Design review of the part built by this model. Coordinates are the model's own, in mm. Give positions to 0.01 mm unless a question says otherwise; leave off trailing zeros. Order: outer loops, then holes, each group sorted by start corner. A loop starts at its lowest first (then second) coordinate and runs counter-clockwise, first axis right, second up.
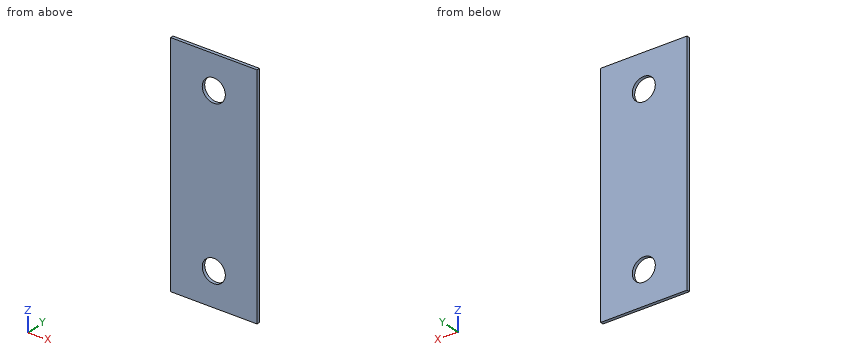
Autodesk Inventor part; units mm, degrees
ref_plane "YZ Plane" through (0, 0, 0) normal (1, 0, 0) x (0, 1, 0)
ref_plane "XZ Plane" through (0, 0, 0) normal (0, 1, 0) x (-1, 0, 0)
ref_plane "XY Plane" through (0, 0, 0) normal (0, 0, 1) x (1, 0, 0)
sketch "Sketch1" plane through (0, 0, 0) normal (0, 1, 0) x (-1, 0, 0)
  line L0 (0, 0) -> (19.05, 0)
  line L1 (19.05, 0) -> (19.05, -50.8)
  line L2 (19.05, -50.8) -> (0, -50.8)
  line L3 (0, -50.8) -> (0, 0)
  line L4 (19.05, 0) -> (0, 0)
  line L5 (0, 0) -> (0, -14.732)
  line L6 (0, -14.732) -> (19.05, -14.732)
  line L7 (19.05, -14.732) -> (19.05, 0)
  line L8 (19.05, -50.8) -> (0, -50.8)
  line L9 (0, -50.8) -> (0, -36.068)
  line L10 (0, -36.068) -> (19.05, -36.068)
  line L11 (19.05, -36.068) -> (19.05, -50.8)
  circle A0 centre (9.525, -7.366) radius 2.54
  circle A1 centre (9.525, -43.434) radius 2.54
  dimension "d0" = 50.8
  dimension "d1" = 19.05
  dimension "d2" = 14.732
  dimension "d3" = 14.732
  dimension "d4" = 5.08
  dimension "d5" = 5.08
extrude "Extrusion1" add sketch "Sketch1" along normal blind 0.7
equation "\"d3\" = d2"
properties part number "Part18.iptMotorProtector2"
1. Take a section at B-B (x = -8). State the section outline as (y, z) points, then the cut area to 3 significant figures.
Recorded:
outline: (0, -50.8) - (0.7, -50.8) - (0.7, -45.47) - (0, -45.47) - close; (0, -41.4) - (0.7, -41.4) - (0.7, -9.4) - (0, -9.4) - close; (0, -5.33) - (0.7, -5.33) - (0.7, 0) - (0, 0) - close
area: 29.9 mm2
2. For line 1 along Z through (x, y) = (-10.25, 0.55); line 2 along Z through (x, y) = (-10.5, 0.3); line 3 along X through (y, z) = (0.2, -5.5), list the stretches that pass through material, from the lowest coordinate up.
Recorded:
line 1: z = -50.8 to -45.87, -41 to -9.8, -4.93 to 0
line 2: z = -50.8 to -45.78, -41.09 to -9.71, -5.02 to 0
line 3: x = -19.05 to -11.25, -7.8 to 0
3. Take a section at A-A (z = -42.5). State the section outline as (x, y) points.
Recorded:
outline: (-19.05, 0) - (-11.89, 0) - (-11.89, 0.7) - (-19.05, 0.7) - close; (-7.16, 0) - (0, 0) - (0, 0.7) - (-7.16, 0.7) - close
4. Take a section at C-C (y = 0.35). State the section outline as (x, z) points (3 decimals).
Recorded:
outline: (-19.05, -50.8) - (0, -50.8) - (0, 0) - (-19.05, 0) - close; hole circle Ø5.08 at (-9.525, -43.434); hole circle Ø5.08 at (-9.525, -7.366)
